Model file for the job. Use its own axes, mm. Face numbers are marked on the shaded views. A direction names the side the tool comes from. Give positions to 0.01 mm unless a question says otherwise; leave off trailing zeros. Write each loop counter-clockwise with the first axis right and the second up, starting at its lowest first coordinate (ties: lowest second). Pieces come first, ordered by that corner, then holes. Notation, with made-up numbers: (42, 28.5) - (77, 28.5) arc R26 cw to (77, 57.5) - close; hole circle Ø5 at (49.25, 13.25). An arc over 180 degrees is marked (long way). One line per item, written item: value. Start each with the question number.
(1) Cut at A-A, the plane z = 12.5. List the corners of the cut face in (x, y).
(2) Drop flat-ended pins along their axis: P1, Ø5, axis at x = -46, z = 3.5, coming from the +Y side; P2, Ø7, axis at x = -23.5, y = -35, coming from the +Z side; P3, Ø3.5, axis at y = 0, z = 2, coming from the -X side; P4, Ø11.5, axis at x = -30, z = 15, coming from the -Y side (3 decimals). Give the stop position or say it passes through.
(3) Cut at D-D, the plane z = 7. List the corners of the cut face in (x, y).
(4) Cut at C-C, the plane x = -36. List the corners of the cut face in (y, z).
(5) Mould opens along Y. For the marked faces 1, 2 and 3 say: pulls with the +Y half, pulls with the -Y half, needs draft (parallel to the pull), parting line crosses it, or undercut.
(6) 3-axis set-ups, long thin cutter, end or side, ignore diameter. For the marked faces 4, 5, 6 and 7: which of +Z, -Z, +X, -X, +Y, -Y reach the whole face in a straight line?
(7) Probe L1, parallel to Y at x = -14, z = 1.95; L2, parallel to Y at x = -38, z = 3.5; L3, parallel to Z at x = -24, y = -3.5. List the from-to ranges inside material, lowest first.
(8) Cut at B-B, the plane y = 5.5. List the corners of the cut face in (x, z).
from build123d import *

# Parameters (mm, degrees)
SKETCH_1_R      = 1.6
EXTRUDE_1_DEPTH = 3
SKETCH_5_W      = 2
SKETCH_5_H      = 3
EXTRUDE_3_DEPTH = 20
EXTRUDE_4_DEPTH = 3


with BuildPart() as part:
    # 草图1 → 凸台-拉伸1 (new body)
    with BuildSketch(Plane.XY):
        Polygon((-10, 10), (-40, 10), (-40, -7), (-80, -7), (-80, -23), (-40, -23), (-40, -40), (-10, -40), align=None)
        with Locations((-14, -35.5)):
            Circle(SKETCH_1_R, mode=Mode.SUBTRACT)
        with Locations((-36, 5.5)):
            Circle(SKETCH_1_R, mode=Mode.SUBTRACT)
        with Locations((-36, -35.5)):
            Circle(SKETCH_1_R, mode=Mode.SUBTRACT)
        with Locations((-14, 5.5)):
            Circle(SKETCH_1_R, mode=Mode.SUBTRACT)
    extrude(amount=EXTRUDE_1_DEPTH)

    # 草图5 → 凸台-拉伸3 (add)
    with BuildSketch(Plane.XY.offset(3)):
        with Locations((-79, -21.5)):
            Rectangle(SKETCH_5_W, SKETCH_5_H)
        with Locations((-79, -8.5)):
            Rectangle(SKETCH_5_W, SKETCH_5_H)
    extrude(amount=EXTRUDE_3_DEPTH)

    # 草图7 → 凸台-拉伸4 (add)
    with BuildSketch(Plane(origin=(0, -7, 0), x_dir=(1, 0, 0), z_dir=(0, 1, 0))):
        Polygon((-78, -23), (-10, -3), (-40, -3), (-40, 0), (-80, 0), (-80, -23), align=None)
    extrude_4 = extrude(amount=EXTRUDE_4_DEPTH)

    # 镜向1: 凸台-拉伸4 across plane
    add(extrude_4.mirror(Plane(origin=(0, -15, 0), x_dir=(0, 0, 1), z_dir=(0, -1, 0))))


solid = part.part
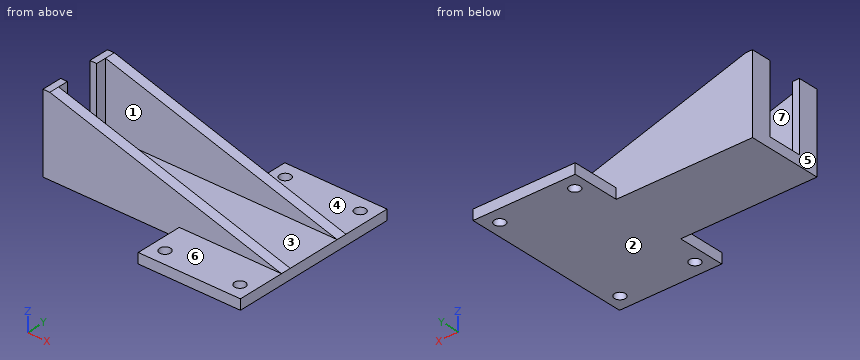
Answers follow:
1. outline: (-80, -26) - (-42.3, -26) - (-42.3, -23) - (-78, -23) - (-78, -20) - (-80, -20) - close; (-80, -10) - (-78, -10) - (-78, -7) - (-42.3, -7) - (-42.3, -4) - (-80, -4) - close
2. P1: stops at y = -4
2. P2: stops at z = 3
2. P3: stops at x = -40
2. P4: passes through
3. outline: (-80, -26) - (-23.6, -26) - (-23.6, -23) - (-78, -23) - (-78, -20) - (-80, -20) - close; (-80, -10) - (-78, -10) - (-78, -7) - (-23.6, -7) - (-23.6, -4) - (-80, -4) - close
4. outline: (-40, 0) - (-37.1, 0) - (-37.1, 3) - (-40, 3) - close; (-33.9, 0) - (3.9, 0) - (3.9, 3) - (-4, 3) - (-4, 10.65) - (-7, 10.65) - (-7, 3) - (-23, 3) - (-23, 10.65) - (-26, 10.65) - (-26, 3) - (-33.9, 3) - close; (7.1, 0) - (10, 0) - (10, 3) - (7.1, 3) - close
5. face 1: undercut
5. face 2: needs draft
5. face 3: undercut
6. face 4: +Z, +X, -X, +Y
6. face 5: +Z, -Z, -X, +Y, -Y
6. face 6: +Z, +X, -X, -Y
6. face 7: +Z, +X
7. L1: y = -40 to -37.1, -33.9 to 3.9, 7.1 to 10
7. L2: y = -26 to -23, -7 to -4
7. L3: z = 0 to 3
8. outline: (-40, 0) - (-37.6, 0) - (-37.6, 3) - (-40, 3) - close; (-34.4, 0) - (-15.6, 0) - (-15.6, 3) - (-34.4, 3) - close; (-12.4, 0) - (-10, 0) - (-10, 3) - (-12.4, 3) - close
